Job drawing, mm, ordinate dimensions from the low corner. One solid piece. Give positions to 0.01 mm unless a question says otherwise; leave off trailing zeros. Order: outer loops, then holes, each group sorted by start corner. A loop starts at its lowest first (then second) coordinate and runs counter-clockwise, first axis right, second up. Notation, with made-up numbers: M -7,70.5 L 2,70.5 A14 cw 2,93.5 Z; hole C -25,65 d5. An arc over 180 degrees is marked long. Put each result on its own line as item: value. Start each with the question number.
1) Drill centre lines: line 1 (Y direction, x = 170, z = 2.5); line 2 (X direction, y = 10.5, z = 0.5). Where is each one in solid material? Low to high. Write a range as [from, to].
2) Pin check, flat tips, straight feed: pin 1 (1.9 mm diameter, centred on x = 135, z = 4.5, fed in from -Y); pin 2 (3 mm diameter, centred on y = 72.5, z = 2.5, fed in from -X); pin 3 (3 mm diameter, centred on x = 44, z = 3.5, fed in from -Y). Stop position of each tip, or through.
3) Cut at A-A (y = 55). Write the cut outline in (x, z), and give its area (3 significant figures).
4) Cut at B-B (x = 49.5). Write the cut outline in (y, z).
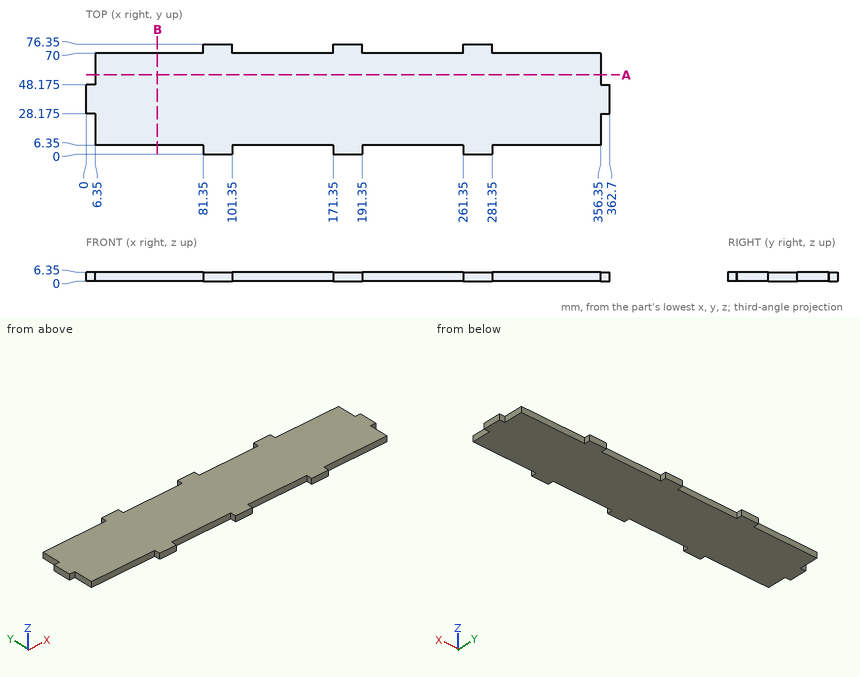
Solution:
1. line 1: [6.35, 70]
1. line 2: [6.35, 356.35]
2. pin 1: y = 6.35
2. pin 2: x = 81.35
2. pin 3: y = 6.35
3. outline: M 6.35,0 L 356.35,0 L 356.35,6.35 L 6.35,6.35 Z
3. area: 2,220 mm²
4. outline: M 6.35,0 L 70,0 L 70,6.35 L 6.35,6.35 Z
